```python
from build123d import *

# Parameters (mm, degrees)
REDONDEO1_R = 5


with BuildPart() as part:
    # Croquis1 → Revolución1 (revolve)
    with BuildSketch(Plane.XY, mode=Mode.PRIVATE) as revoluci_n1_sk:
        Polygon((0, 12.5), (26, 12.5), (26, 10), (30, 10), (30, 16), (6, 16), (0, 14), align=None)
    revolve(revoluci_n1_sk.sketch.rotate(Axis((0, 0, 0), (1, 0, 0)), 90), axis=Axis((0, 0, 0), (1, 0, 0)))

    # Redondeo1
    redondeo1_edges = [part.edges().sort_by_distance(p)[0] for p in [
        (6, 0, -16),
    ]]
    fillet(redondeo1_edges, radius=REDONDEO1_R)


solid = part.part
```
Could you check a few things on this model? Use its own coordinates, in mm. A direction names the side the tool comes from. Coordinates: 2 decimals unless noted, no trailing zeros. Write each loop counter-clockwise with the first axis right and the second up, starting at its lowest first coordinate (ties: lowest second). Pieces come first, ordered by that corner, then holes. Notation, with made-up numbers: (-3, 84) - (6, 84) arc R18 ccw to (6, 94) - close; hole circle Ø10 at (47.25, 38). An arc over 180 degrees is marked (long way). Use a Markdown table: item, result.
Q1. Which directions (+Z, -Z, +X, -X, +Y, -Y) give clear straight access to the entire face, cutting with the end or side of a thin tool? Please do faces 1 (the flat face through (26, -10.2, -0.1)), 2 (the flat face through (30, -0.2, -10.4)).
Geometry check:
| item | result |
|---|---|
| face 1 | -X |
| face 2 | +Z, -Z, +X, +Y, -Y |
Q2. Imagine slicing it at B-B (x = 28). List the corners of the cut face in (y, z) for me, and give its area (3 significant figures).
Geometry check:
| item | result |
|---|---|
| outline | circle Ø32 at (0, 0); hole circle Ø20 at (0, 0) |
| area | 490 mm2 |
Q3. Please list where these lines run through material, in increasing order: L1, parallel to Y at x = 27.45, z = 0; L2, parallel to Z at x = 20.5, y = 9; L3, parallel to X at y = 10.5, z = 3.
Geometry check:
| item | result |
|---|---|
| L1 | y = -16 to -10, 10 to 16 |
| L2 | z = -13.23 to -8.67, 8.67 to 13.23 |
| L3 | x = 26 to 30 |
Q4. Imagine slicing it at A-A (x = 19). List the corners of the cut face in (y, z) for me, and give its area (3 significant figures).
Geometry check:
| item | result |
|---|---|
| outline | circle Ø32 at (0, 0); hole circle Ø25 at (0, 0) |
| area | 313 mm2 |
Q5. I'm going to push flat-ended pins straight in: pin 1 Ø7.5 at (y, z) = (-6, -3.5) entering from -X; pin 2 Ø15 at (y, z) = (0, 0) entering from +X; pin 3 Ø4 at (x, z) = (7, -7) entering from +Y; pin 4 Ø1.5 at (x, z) = (24, -10.5) entering from +Y. Where does each tip first touch, or does it pass through?
Geometry check:
| item | result |
|---|---|
| pin 1 | stops at x = 26 |
| pin 2 | passes through |
| pin 3 | stops at y = 15.2 |
| pin 4 | stops at y = 12.69 |
